Build history of the part. All positions in model axes, mm. A direction names the side the tool comes from. Give positions to 0.01 mm unless a question says otherwise; leave off trailing zeros. Order: outer loops, then holes, each group sorted by start corner. A loop starts at its lowest first (then second) coordinate and runs counter-clockwise, first axis right, second up. Notation, with made-up numbers: (1.25, 3.5) -> (49.25, 3.5) arc R6 cw to (49.25, 7.5) -> close; hole circle Ø10 at (9, -31.5). An arc over 180 degrees is marked (long way). One line per item, written item: value. Start each with the question number.
(1) Probe line 1 (Y direction, x = 69, z = 12); line 2 (Y direction, x = 30, z = 10.25); line 3 (X direction, y = 23.5, z = 7.75). List the from-to ranges inside material, lowest first.
(2) Two-plate mould, pull along Y, no slides. Class faces 1 (the flat face through (40, 2.032, 10)), 2 (the flat face through (38, 0, 6)), 3 (the flat face through (0, 19, 6)): +Y half, -Y half, draft (parallel to the pull), parting line (faces both ways), or undercut.
(3) Saw through at A-A on z = 4.75. Give the cut face in (x, y), plus the area to 3 significant figures.
(4) Pin check, flat tips, straight feed: pin 1 (0.8 mm diameter, centred on y = 25, z = 12, fed in from +X); pin 2 (3 mm diameter, centred on x = 63.5, y = 11, fed in from +Z); pin 3 (0.5 mm diameter, centred on y = 18.5, z = 10.5, fed in from +X). Stop position of each tip, or through.
(5) Saw through at C-C on x = 36. Give the cut face in (y, z).
(6) Which spindle directions (+Z, -Z, +X, -X, +Y, -Y) get a long thin tool onto all of the face, cutting with end or side? Do faces 4 (the flat face through (3.81, 19, 6)), 5 (the flat face through (38, 19, 0)), 6 (the flat face through (38, 38.1, 6)), 7 (the flat face through (41, 34.29, 12)), 8 (the flat face through (40, 3, 11.176)). Say none if no direction does.
(7) Saw through at B-B on y = 27.5. Give the cut face in (x, z), plus the area to 3 significant figures.
```python
from build123d import *

# Parameters (mm, degrees)
SKETCH1_W           = 76.2
SKETCH1_H           = 38.1
BOSS_EXTRUDE1_DEPTH = 12.7
SKETCH3_W           = 34.29
SKETCH3_H           = 30.48
CUT_EXTRUDE1_DEPTH  = 9.652
SKETCH5_W           = 2.54
SKETCH5_H           = 30.48
CUT_EXTRUDE3_DEPTH  = 3.81
SKETCH6_W           = 1.524
SKETCH6_H           = 34.036
CUT_EXTRUDE4_DEPTH  = 73.66


with BuildPart() as part:
    # Sketch1 → Boss-Extrude1 (new body)
    with BuildSketch(Plane.XY):
        with Locations((38.1, 19.05)):
            Rectangle(SKETCH1_W, SKETCH1_H)
    extrude(amount=BOSS_EXTRUDE1_DEPTH)

    # Sketch3 → Cut-Extrude1 (cut)
    with BuildSketch(Plane.XY.offset(12.7)):
        with Locations((20.955, 19.05)):
            Rectangle(SKETCH3_W, SKETCH3_H)
        with Locations((55.245, 19.05)):
            Rectangle(SKETCH3_W, SKETCH3_H)
    extrude(amount=-CUT_EXTRUDE1_DEPTH, mode=Mode.SUBTRACT)

    # Sketch5 → Cut-Extrude3 (cut)
    with BuildSketch(Plane(origin=(76.2, 0, 0), x_dir=(0, 0, -1), z_dir=(1, 0, 0))):
        with Locations((-11.43, 19.05)):
            Rectangle(SKETCH5_W, SKETCH5_H)
    extrude(amount=-CUT_EXTRUDE3_DEPTH, mode=Mode.SUBTRACT)

    # Sketch6 → Cut-Extrude4 (cut)
    with BuildSketch(Plane(origin=(76.2, 0, 0), x_dir=(0, 0, -1), z_dir=(1, 0, 0))):
        with Locations((-10.414, 19.05)):
            Rectangle(SKETCH6_W, SKETCH6_H)
    extrude(amount=-CUT_EXTRUDE4_DEPTH, mode=Mode.SUBTRACT)


solid = part.part
```
Results below:
1. line 1: y = 0 to 3.81, 34.29 to 38.1
1. line 2: y = 0 to 2.03, 36.07 to 38.1
1. line 3: x = 0 to 3.81, 72.39 to 76.2
2. face 1: undercut
2. face 2: -Y half
2. face 3: draft
3. outline: (0, 0) -> (76.2, 0) -> (76.2, 38.1) -> (0, 38.1) -> close; hole (3.81, 3.81) -> (72.39, 3.81) -> (72.39, 34.29) -> (3.81, 34.29) -> close
3. area: 813 mm²
4. pin 1: stops at x = 3.81
4. pin 2: stops at z = 3.05
4. pin 3: stops at x = 2.54
5. outline: (0, 0) -> (38.1, 0) -> (38.1, 12.7) -> (34.29, 12.7) -> (34.29, 11.18) -> (36.07, 11.18) -> (36.07, 9.65) -> (34.29, 9.65) -> (34.29, 3.05) -> (3.81, 3.05) -> (3.81, 9.65) -> (2.03, 9.65) -> (2.03, 11.18) -> (3.81, 11.18) -> (3.81, 12.7) -> (0, 12.7) -> close
6. face 4: +Z
6. face 5: -Z, +X, -X, +Y, -Y
6. face 6: +Z, -Z, +X, -X, +Y
6. face 7: +Z, +X
6. face 8: +X
7. outline: (0, 0) -> (76.2, 0) -> (76.2, 9.65) -> (72.39, 9.65) -> (72.39, 3.05) -> (3.81, 3.05) -> (3.81, 9.65) -> (2.54, 9.65) -> (2.54, 11.18) -> (3.81, 11.18) -> (3.81, 12.7) -> (0, 12.7) -> close
7. area: 292 mm²
